```python
from build123d import *

# Parameters (mm, degrees)
SKETCH1_R              = 25.4
BOSS_EXTRUDE1_DEPTH    = 25.4
CUT_EXTRUDE1_START     = -17.4625
SKETCH2_R              = 25.4
SKETCH2_R_2            = 17.4625
CUT_EXTRUDE1_DEPTH     = 17.4625
CUT_EXTRUDE2_DEPTH     = 44.994090512
F_10_CLEARANCE_HOLE1_D = 5.1054


with BuildPart() as part:
    # Sketch1 → Boss-Extrude1 (new body)
    with BuildSketch(Plane(origin=(0, 0, 0), x_dir=(1, 0, 0), z_dir=(0, 1, 0))):
        with Locations(Location((0, 0, 0), (0, 0, 270))):
            Circle(SKETCH1_R)
    extrude(amount=BOSS_EXTRUDE1_DEPTH)

    # Sketch2 → Cut-Extrude1 (cut)
    with BuildSketch(Plane(origin=(0, 25.4, 0), x_dir=(1, 0, 0), z_dir=(0, 1, 0)).offset(CUT_EXTRUDE1_START)):
        with Locations(Location((0, 0, 0), (0, 0, 270))):
            Circle(SKETCH2_R)
        with Locations(Location((0, 0, 0), (0, 0, 270))):
            Circle(SKETCH2_R_2, mode=Mode.SUBTRACT)
    extrude(amount=CUT_EXTRUDE1_DEPTH, mode=Mode.SUBTRACT)

    # Sketch3 → Cut-Extrude2 (cut, through all)
    with BuildSketch(Plane(origin=(0, 25.4, 0), x_dir=(1, 0, 0), z_dir=(0, 1, 0))):
        with BuildLine():
            ThreePointArc((1.5875, 6.148361062), (0, 6.35), (-1.5875, 6.148361062))
            Line((-1.5875, 6.148361062), (1.5875, 6.148361062))
        make_face()
        with BuildLine():
            Line((1.5875, 6.148361062), (-1.5875, 6.148361062))
            ThreePointArc((-1.5875, 6.148361062), (-3.888564967, -5.020115786), (6.35, 0))
            ThreePointArc((6.35, 0), (5.020115786, 3.888564967), (1.5875, 6.148361062))
        make_face()
        with BuildLine():
            Line((-1.5875, 7.735861062), (-1.5875, 6.148361062))
            ThreePointArc((-1.5875, 6.148361062), (0, 6.35), (1.5875, 6.148361062))
            Line((1.5875, 6.148361062), (1.5875, 7.735861062))
            Line((1.5875, 7.735861062), (-1.5875, 7.735861062))
        make_face()
    extrude(amount=-CUT_EXTRUDE2_DEPTH, mode=Mode.SUBTRACT)

    # #10 Clearance Hole1 (through all)
    with Locations(Plane(origin=(21.082, 7.9375, 0), x_dir=(0, 0, 1), z_dir=(0, 1, 0))):
        with Locations((0, 0), (-18.257547563, -10.541), (-18.257547563, -31.623), (0, -42.164), (18.257547563, -31.623), (18.257547563, -10.541)):
            Hole(F_10_CLEARANCE_HOLE1_D / 2)


solid = part.part
```
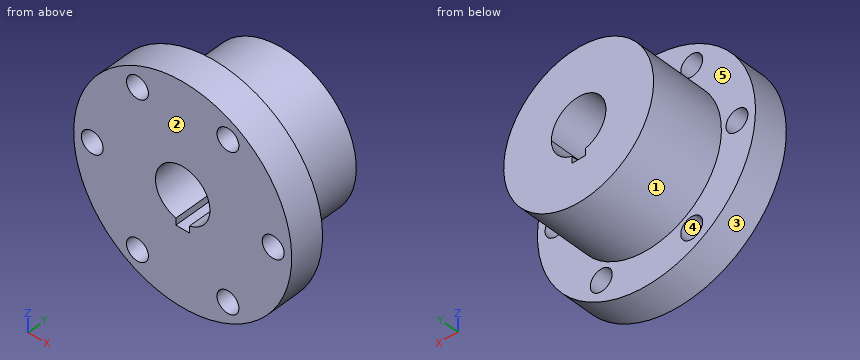
The model under review builds one solid part; all positions refer to its coordinate system, in mm. Face numbers are marked on the shaded views. A direction names the side the tool comes from. Give positions to 0.01 mm unless a question says otherwise; leave off trailing zeros. Write each loop counter-clockwise with the first axis right and the second up, starting at its lowest first coordinate (ties: lowest second). Pieces come first, ordered by that corner, then holes. Notation, with made-up numbers: M 16,57.25 L 68,57.25 A22 ccw 68,78.25 Z; hole C 49.5,14.5 d1. An arc over 180 degrees is marked long. Write item = value, one per line. Start each with the question number.
Q1. We need section C-C (z = -5.5). State the section outline as (x, y) points.
Q2. We need section A-A (x = 0). State the section outline as (y, z) points.
Q3. Mouldability with a two-part tool opening along Z and no side actions: class the marked faces 3, 4 and 5 as released by +Z, released by -Z, zero draft, split by the parting line, or undercut.
Q4. For line 1 (Y direction, x = 22, z = -12); line 2 (X direction, y = 6.25, z = 4.5); line 3 (Z direction, x = -5, y = 23), list the stretches that pass through material, from the lowest coordinate up.
Q5. Clearance check with flat-ended pins moving along their axes: pin 1 (0.8 mm diameter, centred on y = 15, z = -7, fed in from -X); pin 2 (2 mm diameter, centred on y = 19, z = 17, fed in from -X); pin 3 (0.8 mm diameter, centred on y = 15.5, z = -7, fed in from +X); pin 4 (4.5 mm diameter, centred on x = -21.082, z = 0, fed in from +Y). State where each tip first meets the part, or that it passes through.
Q6. We need section D-D (y = 3.5). State the section outline as (x, z) points, plus the area to 3 significant figures.
Q7. Machinability: for the marked faces 1 and 2, which of the approach directions +Z, -Z, +X, -X, +Y, -Y give a long, thin tool a straight path to every point of the face, cutting with its end or side? Answer none if there is none.
Result set:
q1.outline = M -24.8,0 L -3.17,0 L -3.17,25.4 L -16.57,25.4 L -16.57,7.94 L -24.8,7.94 Z; M 3.17,0 L 24.8,0 L 24.8,7.94 L 16.57,7.94 L 16.57,25.4 L 3.17,25.4 Z
q2.outline = M 0,-25.4 L 7.94,-25.4 L 7.94,-17.46 L 25.4,-17.46 L 25.4,-7.74 L 0,-7.74 Z; M 0,6.35 L 25.4,6.35 L 25.4,17.46 L 7.94,17.46 L 7.94,25.4 L 0,25.4 Z
q3.face_3 = split by the parting line
q3.face_4 = undercut
q3.face_5 = zero draft
q4.line_1 = 0 to 7.94
q4.line_2 = -25 to -4.48, 4.48 to 25
q4.line_3 = -16.73 to -3.91, 3.91 to 16.73
q5.pin_1 = -16.17
q5.pin_2 = -7
q5.pin_3 = 16.17
q5.pin_4 = through
q6.outline = C 0,0 d50.8; hole C -21.08,0 d5.11; hole C -10.54,-18.26 d5.11; hole C -10.54,18.26 d5.11; hole M -1.59,-7.74 L 1.59,-7.74 L 1.59,-6.15 A6.35 ccw long -1.59,-6.15 Z; hole C 10.54,-18.26 d5.11; hole C 10.54,18.26 d5.11; hole C 21.08,0 d5.11
q6.area = 1,770 mm2
q7.face_1 = +Y
q7.face_2 = +Z, -Z, +X, -X, -Y
